Build history of the part. All positions in model axes, mm. A direction names the side the tool comes from. Round coordinates to 2 decimals unless told otherwise and drop trailing zeros. Write each loop counter-clockwise with the first axis right and the second up, starting at its lowest first coordinate (ties: lowest second). Pieces come first, ordered by that corner, then holes.
1) Saw through at D-D (y = 1.85). Write the cut outline in (x, z).
2) Saw through at A-A (x = -14). Write the cut outline in (y, z).
3) Saw through at B-B (z = 5). Write the cut outline in (x, y).
4) Which spindle directions (+Z, -Z, +X, -X, +Y, -Y) get a long thin tool onto all of the face, cutting with end or side? Do faces 4 (the flat face through (0, 0, -7)), 5 (the flat face through (0, 1, 6.2)). Say none if no direction does.
5) Pull direction Z, two halves, no side cores. Call faces 1 (the cylindrical face through (-12.76, 1.48, -0.16)), 2 (the flat face through (0, 1, 10)), 3 (the flat face through (0, 3, -7)): +Z half, -Z half, draft (parallel to the pull), parting line (faces both ways), or undercut.
6) Wall check: probe 1 along X at (y, z) = (1.85, 0); probe 2 along Z at (x, y) = (3.5, 2); probe 3 along X at (y, z) = (2.25, 2.25). Give the ranges that are in metal, low to high.
7) Saw through at C-C (z = 0). Write the cut outline in (x, y).
8) Flat gauge pin, fed straight in: pin 1 (2 mm diameter, centred on x = -14, z = 0, fed in from -Y). Where does the tip first touch, or does it go through?
from build123d import *

# Parameters (mm, degrees)
CROQUIS1_W              = 45
CROQUIS1_H              = 20
CROQUIS1_R              = 1.25
CROQUIS1_W_2            = 23.6
CROQUIS1_H_2            = 12.4
SALIENTE_EXTRUIR1_DEPTH = 3


with BuildPart() as part:
    # Croquis1 → Saliente-Extruir1 (new body)
    with BuildSketch(Plane(origin=(0, 0, 0), x_dir=(1, 0, 0), z_dir=(0, 1, 0))):
        Rectangle(CROQUIS1_W, CROQUIS1_H)
        with Locations(Location((14, 0, 0), (0, 0, 270))):
            Circle(CROQUIS1_R, mode=Mode.SUBTRACT)
        with Locations(Location((-14, 0, 0), (0, 0, 270))):
            Circle(CROQUIS1_R, mode=Mode.SUBTRACT)
        Rectangle(CROQUIS1_W_2, CROQUIS1_H_2, mode=Mode.SUBTRACT)
    extrude(amount=SALIENTE_EXTRUIR1_DEPTH)


solid = part.part
Evaluation:
1. outline: (-22.5, -10) - (22.5, -10) - (22.5, 10) - (-22.5, 10) - close; hole circle Ø2.5 at (-14, 0); hole (-11.8, -6.2) - (11.8, -6.2) - (11.8, 6.2) - (-11.8, 6.2) - close; hole circle Ø2.5 at (14, 0)
2. outline: (0, -10) - (3, -10) - (3, -1.25) - (0, -1.25) - close; (0, 1.25) - (3, 1.25) - (3, 10) - (0, 10) - close
3. outline: (-22.5, 0) - (-11.8, 0) - (-11.8, 3) - (-22.5, 3) - close; (11.8, 0) - (22.5, 0) - (22.5, 3) - (11.8, 3) - close
4. face 4: +Z, -Z, +X, -X, -Y
4. face 5: +Y, -Y
5. face 1: undercut
5. face 2: +Z half
5. face 3: draft
6. probe 1: x = -22.5 to -15.25, -12.75 to -11.8, 11.8 to 12.75, 15.25 to 22.5
6. probe 2: z = -10 to -6.2, 6.2 to 10
6. probe 3: x = -22.5 to -11.8, 11.8 to 22.5
7. outline: (-22.5, 0) - (-15.25, 0) - (-15.25, 3) - (-22.5, 3) - close; (-12.75, 0) - (-11.8, 0) - (-11.8, 3) - (-12.75, 3) - close; (11.8, 0) - (12.75, 0) - (12.75, 3) - (11.8, 3) - close; (15.25, 0) - (22.5, 0) - (22.5, 3) - (15.25, 3) - close
8. pin 1: passes through
